from build123d import *

# Parameters (mm, degrees)
SKIZZE1_W                            = 24
SKIZZE1_H                            = 21
AUFSATZ_LINEAR_AUSTRAGEN1_DEPTH      = 10
SKIZZE2_R                            = 2.1
SCHNITT_LINEAR_AUSTRAGEN1_DEPTH      = 20
SCHNITT_LINEAR_AUSTRAGEN1_DEPTH_BACK = 20
SKIZZE3_R                            = 2.1
SCHNITT_LINEAR_AUSTRAGEN2_DEPTH      = 20
SCHNITT_LINEAR_AUSTRAGEN2_DEPTH_BACK = 20
SKIZZE4_R                            = 6
SCHNITT_LINEAR_AUSTRAGEN3_DEPTH      = 10
VERRUNDUNG1_R                        = 1
VERRUNDUNG2_R                        = 1
FASE1_SIZE                           = 0.5


with BuildPart() as part:
    # Skizze1 → Aufsatz-Linear austragen1 (new body)
    with BuildSketch(Plane(origin=(0, 0, 0), x_dir=(1, 0, 0), z_dir=(0, 1, 0))):
        Rectangle(SKIZZE1_W, SKIZZE1_H)
    extrude(amount=AUFSATZ_LINEAR_AUSTRAGEN1_DEPTH)

    # Skizze2 → Schnitt-Linear austragen1 (cut, two sides)
    with BuildSketch(Plane(origin=(0, 0, 0), x_dir=(0, 0, -1), z_dir=(1, 0, 0))) as schnitt_linear_austragen1_sk:
        with Locations((0, 5)):
            Circle(SKIZZE2_R)
    extrude(amount=SCHNITT_LINEAR_AUSTRAGEN1_DEPTH, mode=Mode.SUBTRACT)
    extrude(schnitt_linear_austragen1_sk.sketch, amount=-SCHNITT_LINEAR_AUSTRAGEN1_DEPTH_BACK, mode=Mode.SUBTRACT)

    # Skizze3 → Schnitt-Linear austragen2 (cut, two sides)
    with BuildSketch(Plane.XY) as schnitt_linear_austragen2_sk:
        with Locations((0, 5)):
            Circle(SKIZZE3_R)
    extrude(amount=SCHNITT_LINEAR_AUSTRAGEN2_DEPTH, mode=Mode.SUBTRACT)
    extrude(schnitt_linear_austragen2_sk.sketch, amount=-SCHNITT_LINEAR_AUSTRAGEN2_DEPTH_BACK, mode=Mode.SUBTRACT)

    # Skizze4 → Schnitt-Linear austragen3 (cut)
    with BuildSketch(Plane(origin=(0, 10, 0), x_dir=(-1, 0, 0), z_dir=(0, 1, 0))):
        with Locations((12, -10.5)):
            Circle(SKIZZE4_R)
        with Locations((-12, -10.5)):
            Circle(SKIZZE4_R)
        with Locations((-12, 10.5)):
            Circle(SKIZZE4_R)
        with Locations((12, 10.5)):
            Circle(SKIZZE4_R)
    extrude(amount=-SCHNITT_LINEAR_AUSTRAGEN3_DEPTH, mode=Mode.SUBTRACT)

    # Verrundung1
    verrundung1_edges = [part.edges().sort_by_distance(p)[0] for p in [
        (-6, 5, -10.5),
        (-12, 5, -4.5),
        (6, 5, -10.5),
        (12, 5, -4.5),
        (6, 5, 10.5),
        (12, 5, 4.5),
        (-6, 5, 10.5),
        (-12, 5, 4.5),
    ]]
    fillet(verrundung1_edges, radius=VERRUNDUNG1_R)

    # Verrundung2
    verrundung2_edges = [part.edges().sort_by_distance(p)[0] for p in [
        (12, 10, 0),
        (12, 0, 0),
        (0, 0, 10.5),
        (-7.757359313, 0, 6.257359313),
        (-12, 0, 0),
        (-7.757359313, 0, -6.257359313),
        (0, 0, -10.5),
        (7.757359313, 0, -6.257359313),
        (7.757359313, 0, 6.257359313),
        (11.755928946, 0, -4.22645044),
        (5.72645044, 0, -10.255928946),
        (-5.72645044, 0, -10.255928946),
        (-11.755928946, 0, -4.22645044),
        (-11.755928946, 0, 4.22645044),
        (-5.72645044, 0, 10.255928946),
        (5.72645044, 0, 10.255928946),
        (11.755928946, 0, 4.22645044),
        (7.757359313, 10, 6.257359313),
        (-7.757359313, 10, 6.257359313),
        (0, 10, 10.5),
        (7.757359313, 10, -6.257359313),
        (0, 10, -10.5),
        (-7.757359313, 10, -6.257359313),
        (-12, 10, 0),
        (11.755928946, 10, -4.22645044),
        (5.72645044, 10, -10.255928946),
        (-5.72645044, 10, -10.255928946),
        (-11.755928946, 10, -4.22645044),
        (-11.755928946, 10, 4.22645044),
        (-5.72645044, 10, 10.255928946),
        (5.72645044, 10, 10.255928946),
        (11.755928946, 10, 4.22645044),
    ]]
    fillet(verrundung2_edges, radius=VERRUNDUNG2_R)

    # Fase1
    fase1_edges = [part.edges().sort_by_distance(p)[0] for p in [
        (-12, 5, 2.1),
        (12, 5, 2.1),
        (-2.1, 5, -10.5),
        (-2.1, 5, 10.5),
    ]]
    chamfer(fase1_edges, length=FASE1_SIZE)


solid = part.part
The listing builds one solid part. Answer for the finished solid, in the listing's coordinates (mm). Coordinates: 2 decimals unless noted, no trailing zeros. Order: outer loops, then holes, each group sorted by start corner. A loop starts at its lowest first (then second) coordinate and runs counter-clockwise, first axis right, second up. Notation, with made-up numbers: M 52,1.5 L 77,1.5 A14 cw 77,9.5 Z; hole C -2.75,-12.75 d11. An arc over 180 degrees is marked long. Use CSV: the item, a comma, the result in double quotes.
Q1. Section B-B (y = 2) is taken. Determine the outline of the cut face in (x, z), then the cut area to 3 significant figures.
Here are the results:
outline,"M -12,-3.57 A1 ccw -11.14,-4.56 A6 cw -6.06,-9.64 A1 ccw -5.07,-10.5 L 5.07,-10.5 A1 ccw 6.06,-9.64 A6 cw 11.14,-4.56 A1 ccw 12,-3.57 L 12,3.57 A1 ccw 11.14,4.56 A6 cw 6.06,9.64 A1 ccw 5.07,10.5 L -5.07,10.5 A1 ccw -6.06,9.64 A6 cw -11.14,4.56 A1 ccw -12,3.57 Z"
area,"390 mm2"
Q2. Determine the mould class of faces 1 (the flat face through (0, 0, 0)), 2 (the cylindrical face through (11.699, 0.285, -0.05)), 3 (the cylindrical face through (-1.548, 6.419, -6.041)), 4 (the cylindrical face through (-5.734, 5.056, -10.249)) for opening direction X: pulls with the +X half, pulls with the -X half, needs draft (parallel to the pull), parting line crosses it, or undercut.
Here are the results:
face 1,"needs draft"
face 2,"pulls with the +X half"
face 3,"undercut"
face 4,"pulls with the -X half"
Q3. Section C-C (y = 5.5) is taken. Give the number of separate pieces and of enclosed holes in the cut face, then the cut area to 3 significant figures.
Here are the results:
separate pieces,"4"
enclosed holes,"0"
area,"222 mm2"
Q4. Section A-A (x = 3.75) is taken. Determine the outline of the cut face in (y, z), then the cut area to 3 significant figures.
Here are the results:
outline,"M 0,-9.5 A1 ccw 1,-10.5 L 9,-10.5 A1 ccw 10,-9.5 L 10,9.5 A1 ccw 9,10.5 L 1,10.5 A1 ccw 0,9.5 Z; hole C 5,0 d4.2"
area,"195 mm2"
Q5. Straight lines are drawn through the part: L1, parallel to Y at x = 0, z = 4.5; L2, parallel to X at y = 5, z = -2.75; L3, parallel to X at y = 6, z = 4.25. For each, find the intervals that lie inside material, in ascending order.
Here are the results:
L1,"0 to 2.9, 7.1 to 10"
L2,"-12 to -2.1, 2.1 to 12"
L3,"-11.73 to -1.85, 1.85 to 11.73"
